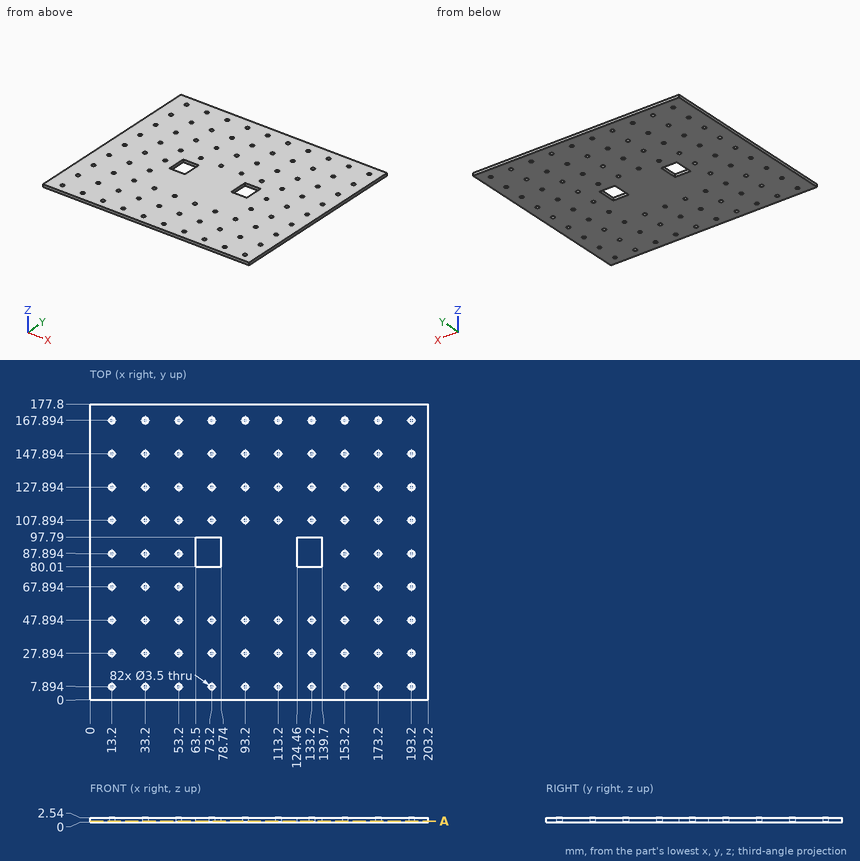
Part print with two shaded views. Sizes in mm from the minimum x, y, z corner. Coordinates: 2 decimals unless noted, no trailing zeros. Answer as a JSON object with one key per item and string values.
Q1. Probe probe 1 along X at (y, z) = (94, 0.3); probe 2 along Y at (x, z) = (136, 1.9). List the from-to ranges inside material, lowest first.
Report:
{"probe 1": "x = 0 to 63.5, 78.74 to 124.46, 139.7 to 203.2", "probe 2": "y = 0 to 80.01, 97.79 to 177.8"}
Q2. Flat gauge pin, fed straight in: P1, Ø3, axis at x = 13.2, y = 47.894, coming from the +Z side. Where does the tip first touch, or does it go through?
Report:
{"P1": "passes through"}
Q3. Cut at A-A (z = 0.6). State how many separate pieces and enclosed holes the cut face has, and give its area (3 significant figures).
Report:
{"separate pieces": "1", "enclosed holes": "84", "area": "34,800 mm2"}
